from build123d import *

# Parameters (mm, degrees)
BOSS_EXTRUDE1_DEPTH                      = 9.5
CBORE_FOR_M12_HEX_HEAD_BOLT3_D           = 6.75
CBORE_FOR_M12_HEX_HEAD_BOLT3_CBORE_D     = 25
CBORE_FOR_M12_HEX_HEAD_BOLT3_CBORE_DEPTH = 5
CUT_EXTRUDE1_DEPTH                       = 19
SKETCH6_3_R                              = 6
SKETCH6_3_R_2                            = 4.785
BOSS_EXTRUDE2_DEPTH                      = 19


with BuildPart() as part:
    # Sketch1 → Boss-Extrude1 (new body, symmetric)
    with BuildSketch(Plane(origin=(0, 0, 0), x_dir=(0, 0, -1), z_dir=(1, 0, 0))):
        with BuildLine():
            Line((12.7, 0), (25.4, 0))
            Line((25.4, 0), (25.4, 19))
            Line((25.4, 19), (-25.4, 19))
            Line((-25.4, 19), (-25.4, 0))
            Line((-25.4, 0), (-12.7, 0))
            ThreePointArc((-12.7, 0), (0, 12.7), (12.7, 0))
        make_face()
    extrude(amount=BOSS_EXTRUDE1_DEPTH, both=True)

    # CBORE for M12 Hex Head Bolt3 (through all)
    with Locations(Plane(origin=(0, 19, 0), x_dir=(1, 0, 0), z_dir=(0, 1, 0))):
        with Locations((0, 19.05), (0, -19.05)):
            CounterBoreHole(CBORE_FOR_M12_HEX_HEAD_BOLT3_D / 2, CBORE_FOR_M12_HEX_HEAD_BOLT3_CBORE_D / 2, CBORE_FOR_M12_HEX_HEAD_BOLT3_CBORE_DEPTH)

    # Sketch6 → Cut-Extrude1 (cut)
    with BuildSketch(Plane(origin=(9.5, 0, 0), x_dir=(0, 0, -1), z_dir=(1, 0, 0))):
        with BuildLine():
            Line((25.4, 2.215), (25.4, 11.785))
            ThreePointArc((25.4, 11.785), (20.615, 7), (25.4, 2.215))
        make_face()
        with BuildLine():
            ThreePointArc((30.185, 7), (28.783505948, 10.383505948), (25.4, 11.785))
            Line((25.4, 11.785), (25.4, 2.215))
            ThreePointArc((25.4, 2.215), (28.783505948, 3.616494052), (30.185, 7))
        make_face()
    extrude(amount=-CUT_EXTRUDE1_DEPTH, mode=Mode.SUBTRACT)

    # Sketch6_3 → Boss-Extrude2 (add)
    with BuildSketch(Plane(origin=(9.5, 0, 0), x_dir=(0, 0, -1), z_dir=(1, 0, 0))):
        with Locations((25.4, 7)):
            Circle(SKETCH6_3_R)
        with Locations((25.4, 7)):
            Circle(SKETCH6_3_R_2, mode=Mode.SUBTRACT)
    extrude(amount=-BOSS_EXTRUDE2_DEPTH)


solid = part.part
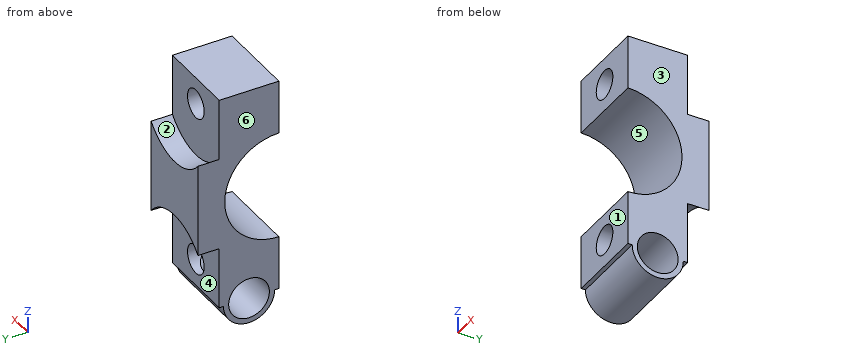
Input: part model. Units: mm. Frame: model coordinates. Face numbers are marked on the shaded views. A direction names the side the tool comes from. Round coordinates to 2 decimals unless told otherwise and drop trailing zeros. Write each loop counter-clockwise with the first axis right and the second up, starting at its lowest first coordinate (ties: lowest second). Pieces come first, ordered by that corner, then holes.
1) Cut plane A-A (x = 0). Count the separate pieces of the cut face and the enclosed holes in it, then the cut area to 3 significant figures.
2) Cut plane C-C (z = 19.05). Return the cut outline in (x, y) (3 decimals), then the cut area to 4 significant figures.
3) Ray query, L1, parallel to Z at x = -0.25, y = 6.75; L2, parallel to X at y = 6.5, z = 19.05 (3 decimals); L3, parallel to Z at x = -8.5, y = 7.75. Return the intervals inside material, ascending.
4) Cut plane B-B (y = 10). Return the cut outline in (x, z) (3 decimals), then the cut area to 3 significant figures.
5) Reachability of the marked faces 1 and 2 from +Z, -Z, +X, -X, +Y, -Y: full face, straight path, thin tool, end or side. Return the list, or none.
6) Contact query for flat-ended pins moving along their axis: P1, Ø0.8, axis at x = 2.5, y = 13.5, coming from the -Z side; P2, Ø9, axis at x = 0, z = 19.05, coming from the +Y side; P3, Ø6, axis at x = -5.5, y = 12, coming from the -Z side. Output: stop coordinate, or through.
7) Cut plane D-D (y = 7). Return the cut outline in (x, z) (3 decimals).
8) Draft query along X for the marked faces 3, 4, 5 and 6. Return one class per face: pulls with the +X half, pulls with the -X half, needs draft (parallel to the pull), parting line crosses it, or undercut.
Geometry says:
1. separate pieces: 3
1. enclosed holes: 1
1. area: 341 mm2
2. outline: (-9.5, 0) - (-3.375, 0) - (-3.375, 14) - (-9.5, 14) - close; (3.375, 0) - (9.5, 0) - (9.5, 14) - (3.375, 14) - close
2. area: 171.5 mm2
3. L1: z = -31.39 to -30.18, -20.62 to -19.41, -15.68 to -10.76, 10.76 to 15.68, 22.42 to 25.4
3. L2: x = -9.5 to -3.375, 3.375 to 9.5
3. L3: z = -31.35 to -30.13, -20.67 to -10.06, 10.06 to 25.4
4. outline: (-9.5, -30.596) - (9.5, -30.596) - (9.5, -29.128) - (-9.5, -29.128) - close; (-9.5, -21.672) - (9.5, -21.672) - (9.5, -7.829) - (-9.5, -7.829) - close; (-9.5, 7.829) - (9.5, 7.829) - (9.5, 25.4) - (-9.5, 25.4) - close; hole circle Ø6.75 at (0, 19.05); hole (-3.172, -20.204) - (3.172, -20.204) arc R3.375 ccw (long way) to start
4. area: 563 mm2
5. face 1: +Z, -Z, +X, -X, -Y
5. face 2: +Z, +Y
6. P1: stops at z = -25.4
6. P2: stops at y = 14
6. P3: stops at z = -31.06
7. outline: (-9.5, -31.4) - (9.5, -31.4) - (9.5, -30.185) - (-9.5, -30.185) - close; (-9.5, -20.615) - (9.5, -20.615) - (9.5, -10.597) - (-9.5, -10.597) - close; (-9.5, 10.597) - (9.5, 10.597) - (9.5, 25.4) - (-9.5, 25.4) - close; hole circle Ø6.75 at (0, 19.05); hole (-3.357, -19.4) - (3.357, -19.4) arc R3.375 ccw (long way) to start
8. face 3: pulls with the +X half
8. face 4: undercut
8. face 5: needs draft
8. face 6: pulls with the -X half
